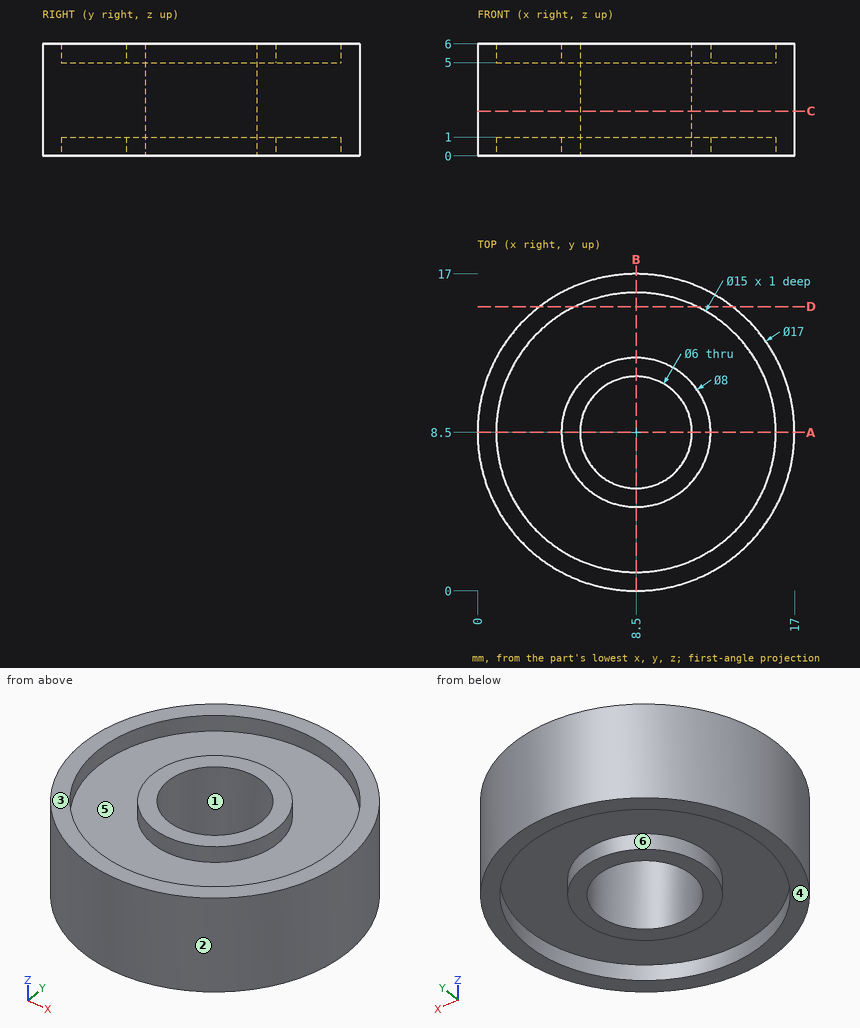
Input: dimensioned drawing with shaded views. Units: mm. Origin: part minimum x, y, z. A direction names the side the tool comes from. Round coordinates to 2 decimals unless told otherwise and drop trailing zeros. Write each loop counter-clockwise with the first axis right and the second up, starting at its lowest first coordinate (ties: lowest second). Pieces come first, ordered by that corner, then holes. Notation, with made-up numbers: (64.25, 88) - (109.25, 88) arc R29 ccw to (109.25, 123) - close; hole circle Ø7 at (27, 0). An arc over 180 degrees is marked (long way). Write item = value, one per line.
(1) Access query for the marked faces 4, 5 and 6. Directions: +Z, -Z, +X, -X, +Y, -Y. A direction counts if a zero-diameter tool reaches every point of the face in a straight line with its end or side. Return the directions, or none.
Geometry check:
face_4 = -Z, +X, -X, +Y, -Y
face_5 = +Z
face_6 = -Z
(2) Contact query for flat-ended pins moving along their axis: pin 1 Ø1 at (x, z) = (3.5, 4.5) entering from +Y; pin 2 Ø1.5 at (x, z) = (14, 1.5) entering from +Y; pin 3 Ø5 at (x, y) = (8.5, 8.5) entering from -Z; pin 4 Ø1.5 at (x, z) = (15, 2) entering from -Y. Output: stop coordinate, or through.
Geometry check:
pin_1 = 15.71
pin_2 = 15.55
pin_3 = through
pin_4 = 2.24
(3) Section query D-D on y = 15.25. Output: boundary loops of the cut face in (x, z).
Geometry check:
outline = (3.33, 0) - (5.23, 0) - (5.23, 1) - (11.77, 1) - (11.77, 0) - (13.67, 0) - (13.67, 6) - (11.77, 6) - (11.77, 5) - (5.23, 5) - (5.23, 6) - (3.33, 6) - close
(4) Section query C-C on z = 2.4. Output: boundary loops of the cut face in (x, y), then the cut area to 3 significant figures.
Geometry check:
outline = circle Ø17 at (8.5, 8.5); hole circle Ø6 at (8.5, 8.5)
area = 199 mm^2
(5) Material intervals for probe 1 along Y at (x, z) = (8.5, 5.5); probe 2 along Y at (x, z) = (6.5, 0.6); probe 3 along Y at (x, z) = (1, 4.8), sorted ascending.
Geometry check:
probe_1 = 0 to 1, 4.5 to 5.5, 11.5 to 12.5, 16 to 17
probe_2 = 0.24 to 1.27, 5.04 to 6.26, 10.74 to 11.96, 15.73 to 16.76
probe_3 = 4.5 to 12.5
(6) Section query A-A on y = 8.5. Output: boundary loops of the cut face in (x, z).
Geometry check:
outline = (0, 0) - (1, 0) - (1, 1) - (4.5, 1) - (4.5, 0) - (5.5, 0) - (5.5, 6) - (4.5, 6) - (4.5, 5) - (1, 5) - (1, 6) - (0, 6) - close; (11.5, 0) - (12.5, 0) - (12.5, 1) - (16, 1) - (16, 0) - (17, 0) - (17, 6) - (16, 6) - (16, 5) - (12.5, 5) - (12.5, 6) - (11.5, 6) - close
(7) Pull-direction query (X, two-part tool) for the marked faces 1, 2 and 3; classes: +X half, -X half, draft (parallel to the pull), parting line (faces both ways), or undercut.
Geometry check:
face_1 = undercut
face_2 = parting line
face_3 = draft
